Answer from the drawing. Dimensions are ordinates in mm from the lowest x, y and z of the part. Coordinates: 2 decimals unless noted, no trailing zeros. Order: outer loops, then holes, each group sorted by start corner. A loop starts at its lowest first (then second) coordinate and runs counter-clockwise, first axis right, second up. Notation, with made-up numbers: (46.5, 19) -> (85.5, 19) arc R23 cw to (85.5, 36) -> close; hole circle Ø5 at (-34.5, 56). An arc over 180 degrees is marked (long way). Answer as a JSON object with one key per item and string values. Group by question number.
1) Given pin 1 (0.9 mm diameter, centred on x = 51.5, y = 1.5, fed in from -Z); pin 2 (1 mm diameter, centred on x = 71, y = 0.5, fed in from -Z), each flat-ended and moving along its own axis, determine where each tip first touches the part or whether it passes through.
2) Section B-B on y = 2.4 is taken. Determine the outline of the cut face in (x, z), and give its area (3 significant figures).
3) Section D-D on x = 101 is taken. Determine the outline of the cut face in (y, z).
4) Section A-A on z = 89.5 is taken. Determine the outline of the cut face in (x, y).
5) Consider L1, parallel to X at y = 2.55, z = 116.5; L2, parallel to X at y = 2.7, z = 128; L3, parallel to Z at x = 51.5, y = 2.55. Determine where each line is inside the solid, lowest interval first.
6) Section C-C on x = 69 is taken. Determine the outline of the cut face in (y, z), and give its area (3 significant figures).
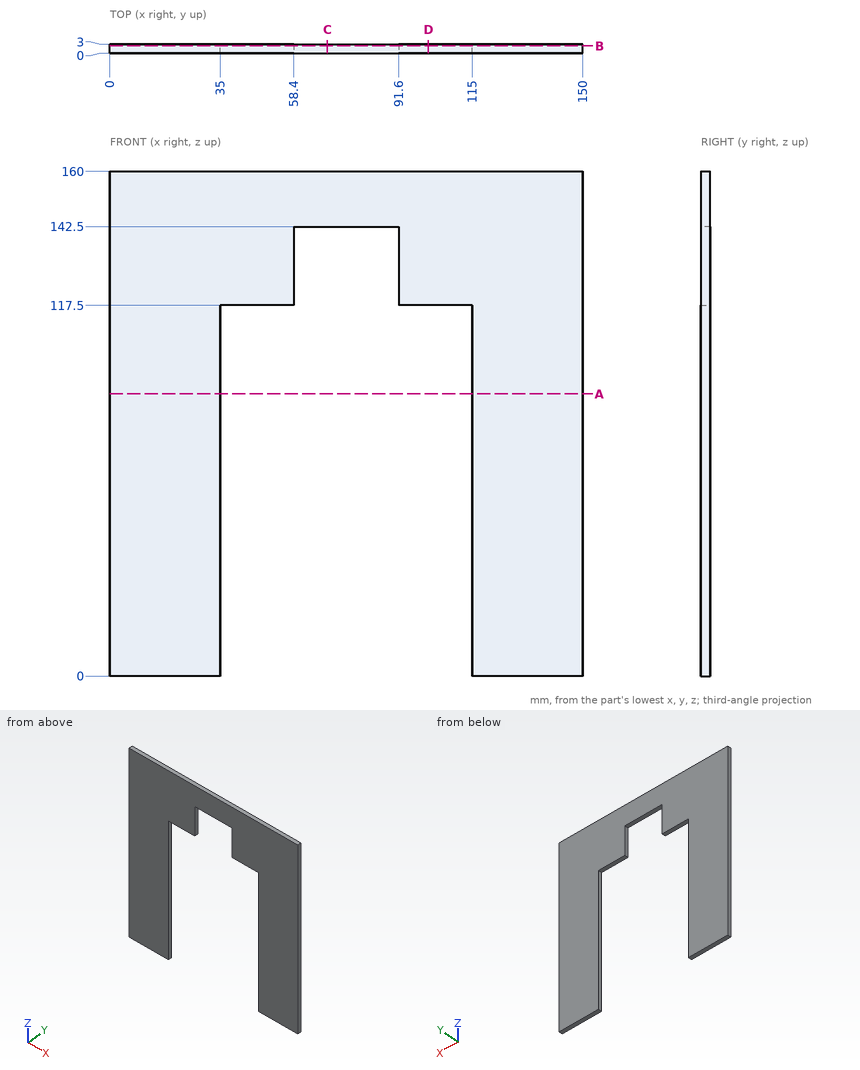
Worked answers:
{
 "1": {"pin 1": "stops at z = 117.5", "pin 2": "stops at z = 142.5"},
 "2": {"outline": "(0, 0) -> (35, 0) -> (35, 117.5) -> (58.4, 117.5) -> (58.4, 142.5) -> (91.6, 142.5) -> (91.6, 117.5) -> (115, 117.5) -> (115, 0) -> (150, 0) -> (150, 160) -> (0, 160) -> close", "area": "13,800 mm²"},
 "3": {"outline": "(0, 117.5) -> (3, 117.5) -> (3, 160) -> (0, 160) -> close"},
 "4": {"outline": "(0, 0) -> (35, 0) -> (35, 3) -> (0, 3) -> close; (115, 0) -> (150, 0) -> (150, 3) -> (115, 3) -> close"},
 "5": {"L1": "x = 0 to 35, 115 to 150", "L2": "x = 0 to 58.4, 91.6 to 150", "L3": "z = 117.5 to 160"},
 "6": {"outline": "(0, 142.5) -> (3, 142.5) -> (3, 160) -> (0, 160) -> close", "area": "52.5 mm²"}
}
